Build history of the part. All positions in model axes, mm. Give positions to 0.01 mm unless a question says otherwise; leave off trailing zeros. Write each loop counter-clockwise with the first axis right and the second up, starting at its lowest first coordinate (ties: lowest second). Pieces come first, ordered by that corner, then holes. Notation, with made-up numbers: M 15,66 L 67,66 A7 ccw 67,70 Z; hole C 76.25,64 d3. An arc over 180 degrees is marked long. Return JSON: item names as keys, results as strings. Group by question number.
Q1. Band-saw the part on C-C, the plane z = 0. Give the cut face in (x, y), then the cut area to 3 significant figures.
Q2. Band-saw the part on B-B, the plane x = -17.5. Give the cut face in (y, z) (3 decimals).
Q3. Band-saw the part on D-D, the plane y = 4.25. Count the separate pieces of the cut face and the enclosed holes in it, then the cut area to 3 significant figures.
Q4. Flat gauge pins, fed straight in: pin 1 Ø3 at (x, z) = (0, 12.5) entering from -Y; pin 2 Ø3 at (x, z) = (-28.82, 11.15) entering from +Y; pin 3 Ø1.5 at (y, z) = (3.5, -31.5) entering from -X; pin 4 Ø3 at (x, y) = (32, 7) entering from -Z. Where does each tip first touch, or does it go through?
Q5. Wall check: probe 1 along X at (y, z) = (3.75, 0); probe 2 along X at (y, z) = (2, 17.5); probe 3 along X at (y, z) = (6, -36). Give the ranges that are in metal, low to high.
Q6. Band-saw the part on A-A, the plane z = 17.5. Give the cut face in (x, y), then the cut area to 3 significant figures.
Q7. Pull direction X, two halves, no side cores. Call faces 1 (the flat face through (46.079, 3.944, -56.737)), 2 (the cylindrical face through (-3.955, 3.944, -5.158)), 3 (the flat face through (15, 4, 27.025)): +X half, -X half, draft (parallel to the pull), parting line (faces both ways), or undercut.
from build123d import *

# Parameters (mm, degrees)
SKETCH1_R           = 13.5001
SKETCH1_R_2         = 6.5
SKETCH1_R_3         = 2.1
SKETCH1_R_4         = 2.5
SKETCH1_R_5         = 1.25
BOSS_EXTRUDE1_DEPTH = 8.001
FILLET1_R           = 2.5


with BuildPart() as part:
    # Sketch1 → Boss-Extrude1 (new body)
    with BuildSketch(Plane(origin=(0, 0, 0), x_dir=(1, 0, 0), z_dir=(0, 1, 0))):
        with BuildLine():
            Line((-35.1724, 27.25881268), (-35.1724, -27.025))
            Line((-35.1724, -27.025), (65.6524, -27.025))
            Line((65.6524, -27.025), (65.6524, 27.25881268))
            ThreePointArc((65.6524, 27.25881268), (63.355608012, 38.071472897), (56.861869136, 47.016875617))
            Line((56.861869136, 47.016875617), (34.989131558, 66.732353738))
            ThreePointArc((34.989131558, 66.732353738), (32.657534218, 68.162444257), (29.968168585, 68.661260389))
            Line((29.968168585, 68.661260389), (0.511831415, 68.661260389))
            ThreePointArc((0.511831415, 68.661260389), (-2.177534218, 68.162444257), (-4.509131558, 66.732353738))
            Line((-4.509131558, 66.732353738), (-26.381869136, 47.016875617))
            ThreePointArc((-26.381869136, 47.016875617), (-32.875608012, 38.071472897), (-35.1724, 27.25881268))
        make_face()
        with Locations(Location((-8.5725, 27.25881268, 0), (0, 0, 270))):
            Circle(SKETCH1_R, mode=Mode.SUBTRACT)
        with Locations(Location((39.0525, 27.25881268, 0), (0, 0, 270))):
            Circle(SKETCH1_R, mode=Mode.SUBTRACT)
        with Locations(Location((0, 0, 0), (0, 0, 270))):
            Circle(SKETCH1_R_2, mode=Mode.SUBTRACT)
        with Locations(Location((0.511831415, 61.161999075, 0), (0, 0, 270))):
            Circle(SKETCH1_R_3, mode=Mode.SUBTRACT)
        with Locations(Location((29.968168585, 61.161999075, 0), (0, 0, 270))):
            Circle(SKETCH1_R_3, mode=Mode.SUBTRACT)
        with Locations(Location((-28.8224, -11.15, 0), (0, 0, 270))):
            Circle(SKETCH1_R_4, mode=Mode.SUBTRACT)
        with Locations(Location((59.3024, -17.5, 0), (0, 0, 270))):
            Circle(SKETCH1_R_4, mode=Mode.SUBTRACT)
        with Locations(Location((15.24, 58.661260389, 0), (0, 0, 270))):
            Circle(SKETCH1_R_4, mode=Mode.SUBTRACT)
        with Locations(Location((12.5, 0, 0), (0, 0, 270))):
            Circle(SKETCH1_R_5, mode=Mode.SUBTRACT)
        with Locations(Location((0, -12.5, 0), (0, 0, 270))):
            Circle(SKETCH1_R_5, mode=Mode.SUBTRACT)
        with Locations(Location((-12.5, 0, 0), (0, 0, 270))):
            Circle(SKETCH1_R_5, mode=Mode.SUBTRACT)
    extrude(amount=BOSS_EXTRUDE1_DEPTH)

    # Fillet1
    fillet1_edges = [part.edges().sort_by_distance(p)[0] for p in [
        (65.6524, 4.0005, 27.025),
        (-35.1724, 4.0005, 27.025),
    ]]
    fillet(fillet1_edges, radius=FILLET1_R)


solid = part.part
From the geometry:
{
 "1": {"outline": "M -35.17,0 L -13.75,0 L -13.75,8 L -35.17,8 Z; M -11.25,0 L -6.5,0 L -6.5,8 L -11.25,8 Z; M 6.5,0 L 11.25,0 L 11.25,8 L 6.5,8 Z; M 13.75,0 L 65.65,0 L 65.65,8 L 13.75,8 Z", "area": "663 mm^2"},
 "2": {"outline": "M 0,-55.023 L 8.001,-55.023 L 8.001,-37.386 L 0,-37.386 Z; M 0,-17.132 L 8.001,-17.132 L 8.001,27.025 L 0,27.025 Z"},
 "3": {"separate pieces": "1", "enclosed holes": "11", "area": "7,260 mm^2"},
 "4": {"pin 1": "stops at y = 0", "pin 2": "passes through", "pin 3": "stops at x = -34.94", "pin 4": "stops at z = -68.64"},
 "5": {"probe 1": "x = -35.17 to -13.75, -11.25 to -6.5, 6.5 to 11.25, 13.75 to 65.65", "probe 2": "x = -35.17 to 56.8, 61.8 to 65.65", "probe 3": "x = -33.7 to -18.86, 1.72 to 28.76, 49.34 to 64.18"},
 "6": {"outline": "M -35.17,0 L 56.8,0 L 56.8,8 L -35.17,8 Z; M 61.8,0 L 65.65,0 L 65.65,8 L 61.8,8 Z", "area": "767 mm^2"},
 "7": {"face 1": "+X half", "face 2": "undercut", "face 3": "draft"}
}
